Geometry: final body of the model. Coordinates: model frame, mm. A direction names the side the tool comes from. Round coordinates to 2 decimals unless told otherwise and drop trailing zeros. Write each loop counter-clockwise with the first axis right and the second up, starting at its lowest first coordinate (ties: lowest second). Pieces come first, ordered by that corner, then holes. Notation, with made-up numbers: M 60.25,71 L 75.25,71 A34 ccw 75.25,102 Z; hole C 49.25,36 d4. An arc over 180 degrees is marked long. Answer as CSV lines item,"result". Start each with the question number.
Q1. Reachability of faces 1 (the flat face through (0, -3, 6)), 2 (the flat face through (0, 0, 7.5)), 3 (the flat face through (-15, 4, 11)), 4 (the flat face through (-14.25, 3, 10)), 5 (the flat face through (-15.75, 1, 7)) from +Z, -Z, +X, -X, +Y, -Y: full face, straight path, thin tool, end or side. Return the list, or none.
Q2. First-contact query: pin 1 (2 mm diameter, centred on x = -5, y = -2.5, fed in from -Z); pin 2 (5.5 mm diameter, centred on x = -12.75, z = 0, fed in from -Y); pin 3 (2.5 mm diameter, centred on x = -2, z = 10, fed in from +Y); pin 4 (8 mm diameter, centred on x = -12, z = 3.5, fed in from -Y). Flat tips, straight axial feed; report the tip coordinate or a pass-through.
Q3. Section query C-C on x = -11.5. Output: boundary loops of the cut face in (y, z).
Q4. Section query B-B on y = -2. Output: boundary loops of the cut face in (x, z), and give its area (3 significant figures).
Q5. Section query A-A on x = 0. Output: boundary loops of the cut face in (y, z).
Q6. Ray query, probe 1 along Z at (x, y) = (-12.75, 1.6); probe 2 along Z at (x, y) = (8.5, -3.75); probe 3 along Z at (x, y) = (-11, 3.75). Return the intervals inside material, ascending.
```python
from build123d import *

# Parameters (mm, degrees)
BOSS_EXTRUDE1_DEPTH  = 5
M3_CLEARANCE_HOLE1_D = 3.4
CUT_EXTRUDE1_DEPTH   = 23.182481827
SKETCH5_W            = 9
SKETCH5_H            = 5
CUT_EXTRUDE2_DEPTH   = 35.077118423
CUT_EXTRUDE5_DEPTH   = 21.422108118
CHAMFER1_SIZE        = 2
FILLET5_R            = 0.5
FILLET6_R            = 1


with BuildPart() as part:
    # Sketch1 → Boss-Extrude1 (new, symmetric)
    with BuildSketch(Plane(origin=(0, 0, 0), x_dir=(1, 0, 0), z_dir=(0, 1, 0))):
        with BuildLine():
            Line((12.75, 3), (-12.75, 3))
            ThreePointArc((-12.75, 3), (-14.871320344, 2.121320344), (-15.75, 0))
            Line((-15.75, 0), (-15.75, -12))
            Line((-15.75, -12), (15.75, -12))
            Line((15.75, -12), (15.75, 0))
            ThreePointArc((15.75, 0), (14.871320344, 2.121320344), (12.75, 3))
        make_face()
    extrude(amount=BOSS_EXTRUDE1_DEPTH, both=True)

    # M3 Clearance Hole1 (through all)
    with Locations(Plane(origin=(0, 5, 0), x_dir=(1, 0, 0), z_dir=(0, 1, 0))):
        with Locations((-12.75, 0), (12.75, 0)):
            Hole(M3_CLEARANCE_HOLE1_D / 2)

    # Sketch4 → Cut-Extrude1 (cut, through all)
    with BuildSketch(Plane(origin=(0, 5, 0), x_dir=(1, 0, 0), z_dir=(0, 1, 0))):
        with BuildLine():
            Line((-12.75, -7.5), (12.75, -7.5))
            ThreePointArc((12.75, -7.5), (14.25, -9), (12.75, -10.5))
            Line((12.75, -10.5), (-12.75, -10.5))
            ThreePointArc((-12.75, -10.5), (-14.25, -9), (-12.75, -7.5))
        make_face()
    extrude(amount=-CUT_EXTRUDE1_DEPTH, mode=Mode.SUBTRACT)

    # Sketch5 → Cut-Extrude2 (cut, through all)
    with BuildSketch(Plane(origin=(15.75, 0, 0), x_dir=(0, 0, -1), z_dir=(1, 0, 0))):
        with Locations((-1.5, -2.5)):
            Rectangle(SKETCH5_W, SKETCH5_H)
    extrude(amount=-CUT_EXTRUDE2_DEPTH, mode=Mode.SUBTRACT)

    # Sketch6 → Cut-Extrude5 (cut, through all)
    with BuildSketch(Plane.XY.offset(9)):
        Polygon((-12.75, 5), (-14.25, 5), (-14.25, 0), (14.25, 0), (14.25, 5), (12.75, 5), align=None)
    extrude(amount=CUT_EXTRUDE5_DEPTH, mode=Mode.SUBTRACT)

    # Chamfer1
    chamfer1_edges = [part.edges().sort_by_distance(p)[0] for p in [
        (-15, 5, 12),
        (15, 5, 12),
    ]]
    chamfer(chamfer1_edges, length=CHAMFER1_SIZE)

    # Fillet5
    fillet5_edges = [part.edges().sort_by_distance(p)[0] for p in [
        (-15, 5, 10),
        (15, 5, 10),
        (15.75, -1, 12),
        (-14.25, 1.5, 12),
        (-15.75, -1, 12),
        (15.75, -2.5, 6),
        (-15.75, -2.5, 6),
        (14.25, 1.5, 12),
    ]]
    fillet(fillet5_edges, radius=FILLET5_R)

    # Fillet6
    fillet6_edges = [part.edges().sort_by_distance(p)[0] for p in [
        (0, 0, 6),
        (-15.603553391, 0, 6.146446609),
        (15.603553391, 0, 6.146446609),
    ]]
    fillet(fillet6_edges, radius=FILLET6_R)


solid = part.part
```
Entries:
1,face 1,"-Z, +X, -X, -Y"
1,face 2,"+Y, -Y"
1,face 3,"+Z, +X, -X, +Y"
1,face 4,"+Z, +Y"
1,face 5,"+Z, -Z, -X, +Y, -Y"
2,pin 1,"stops at z = 6"
2,pin 2,"stops at y = 0"
2,pin 3,"stops at y = 0"
2,pin 4,"stops at y = -5"
3,outline,"M -5,6 L -1,6 A1 cw 0,5 L 0,1.15 L 5,1.15 L 5,7.5 L -5,7.5 Z; M -5,10.5 L 0,10.5 L 0,12 L -5,12 Z; M 0,-3 L 5,-3 L 5,-1.15 L 0,-1.15 Z"
4,outline,"M -15.75,6.5 A0.5 ccw -15.25,6 L 15.25,6 A0.5 ccw 15.75,6.5 L 15.75,11.5 A0.5 ccw 15.25,12 L -15.25,12 A0.5 ccw -15.75,11.5 Z; hole M -12.75,7.5 L 12.75,7.5 A1.5 ccw 12.75,10.5 L -12.75,10.5 A1.5 ccw Z"
4,area,"105 mm^2"
5,outline,"M -5,6 L -1,6 A1 cw 0,5 L 0,-3 L 5,-3 L 5,7.5 L -5,7.5 Z; M -5,10.5 L 0,10.5 L 0,12 L -5,12 Z"
6,probe 1,"z = -3 to -1.7, 1.7 to 7.5"
6,probe 2,"z = 6 to 7.5, 10.5 to 12"
6,probe 3,"z = -3 to 7.5"
